CAD build for the part. Positions are in the model's coordinates, mm. Face numbers are marked on the shaded views. A direction names the side the tool comes from. Coordinates: 2 decimals unless noted, no trailing zeros. Write each loop counter-clockwise with the first axis right and the second up, starting at its lowest first coordinate (ties: lowest second). Pieces come first, ordered by that corner, then holes. Notation, with made-up numbers: (11.5, 39.25) - (29.5, 39.25) arc R33 ccw to (29.5, 71.25) - close; hole circle Ø7 at (39.5, 73.5). An arc over 180 degrees is marked (long way). One line per question, with ' | ' between items. Start each with the question number.
1. Band-saw the part on D-D, the plane z = 42. Write the cut outline in (x, y).
2. Probe line 1 (Z direction, x = -14.5, y = -7.5); line 2 (Z direction, x = 0, y = -11.25); line 3 (Y direction, x = -4, z = 5). List the from-to ranges inside material, lowest first.
3. Which spindle directions (+Z, -Z, +X, -X, +Y, -Y) get a long thin tool onto all of the face, cutting with end or side? Do the marked faces 5, 6 and 7. Say none if no direction does.
4. Flat gauge pin, fed straight in: P1, Ø3, axis at y = 4.5, z = 18.5, coming from the +X side. Where does the tip first touch, or does it go through?
5. Band-saw the part on A-A, the plane y = -3. Write the cut outline in (x, z), then the cut area to 3 significant figures.
6. Band-saw the part on C-C, the plane x = -16. Write the cut outline in (y, z).
7. Two-plate mould, pull along Z, no slides. Class the marked faces 1, 2, 3 and 4: +Z half, -Z half, draft (parallel to the pull), parting line (faces both ways), or undercut.
from build123d import *

# Parameters (mm, degrees)
SKETCH_W        = 50
SKETCH_H        = 50
PAD_DEPTH       = 50
SKETCH001_R     = 7.5
HOLE_DEPTH      = 50.001
SKETCH002_W     = 15
SKETCH002_H     = 15
POCKET_DEPTH    = 50.001
POCKET001_DEPTH = 50.001
FILLET_R        = 5


with BuildPart() as part:
    # Sketch → Pad (new body)
    with BuildSketch(Plane.XY):
        Rectangle(SKETCH_W, SKETCH_H)
    extrude(amount=PAD_DEPTH)

    # Sketch001 (on Face3 of Pad) → Hole (cut, through all)
    with BuildSketch(Plane.XZ.offset(25)):
        with Locations((0, 25)):
            Circle(SKETCH001_R)
    extrude(amount=-HOLE_DEPTH, mode=Mode.SUBTRACT)

    # Sketch002 (on Face4 of Hole) → Pocket (cut, through all)
    with BuildSketch(Plane.XY.offset(50)):
        Rectangle(SKETCH002_W, SKETCH002_H)
    extrude(amount=-POCKET_DEPTH, mode=Mode.SUBTRACT)

    # Sketch003 (on Face5 of Pocket) → Pocket001 (cut, through all)
    with BuildSketch(Plane.YZ.offset(25)):
        Polygon((4.330127, 17.5), (8.660254, 25), (4.330127, 32.5), (-4.330127, 32.5), (-8.660254, 25), (-4.330127, 17.5), align=None)
    extrude(amount=-POCKET001_DEPTH, mode=Mode.SUBTRACT)

    # Fillet
    fillet_edges = [part.edges().sort_by_distance(p)[0] for p in [
        (0, -25, 50),
        (-25, 0, 50),
        (0, 25, 50),
        (25, 0, 50),
        (25, 25, 25),
        (25, -25, 25),
        (-25, -25, 25),
        (0, -25, 0),
        (25, 0, 0),
        (-25, 0, 0),
        (0, 25, 0),
        (-25, 25, 25),
    ]]
    fillet(fillet_edges, radius=FILLET_R)


solid = part.part
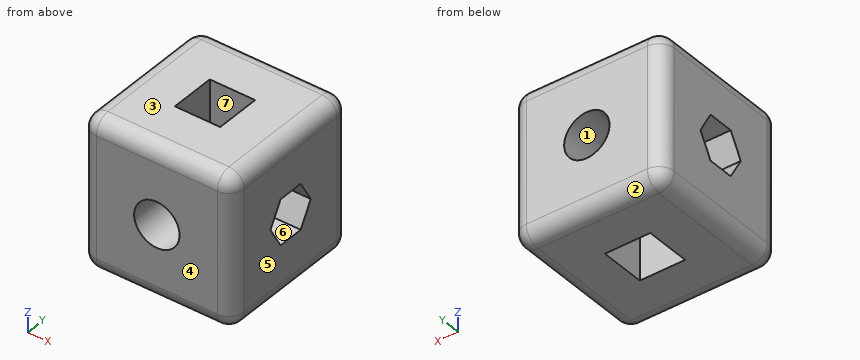
Filled in:
1) outline: (-25, -20) arc R5 ccw to (-20, -25) - (20, -25) arc R5 ccw to (25, -20) - (25, 20) arc R5 ccw to (20, 25) - (-20, 25) arc R5 ccw to (-25, 20) - close; hole (-7.5, -7.5) - (7.5, -7.5) - (7.5, 7.5) - (-7.5, 7.5) - close
2) line 1: z = 0 to 22.99, 27.01 to 50 | line 2: z = 0 to 17.5, 32.5 to 50 | line 3: y = -25 to -7.5, 7.5 to 25
3) face 5: +Z, -Z, +X, +Y, -Y | face 6: +X, -X | face 7: +Z, -Z
4) P1: stops at x = 25
5) outline: (-25, 5) arc R5 ccw to (-20, 0) - (-7.5, 0) - (-7.5, 17.5) - (-25, 17.5) - close; (-25, 32.5) - (-7.5, 32.5) - (-7.5, 50) - (-20, 50) arc R5 ccw to (-25, 45) - close; (7.5, 0) - (20, 0) arc R5 ccw to (25, 5) - (25, 17.5) - (7.5, 17.5) - close; (7.5, 32.5) - (25, 32.5) - (25, 45) arc R5 ccw to (20, 50) - (7.5, 50) - close | area: 1,200 mm²
6) outline: (-25, 5) arc R5 ccw to (-20, 0) - (20, 0) arc R5 ccw to (25, 5) - (25, 45) arc R5 ccw to (20, 50) - (-20, 50) arc R5 ccw to (-25, 45) - close; hole (-8.66, 25) - (-4.33, 17.5) - (4.33, 17.5) - (8.66, 25) - (4.33, 32.5) - (-4.33, 32.5) - close
7) face 1: undercut | face 2: -Z half | face 3: +Z half | face 4: draft
